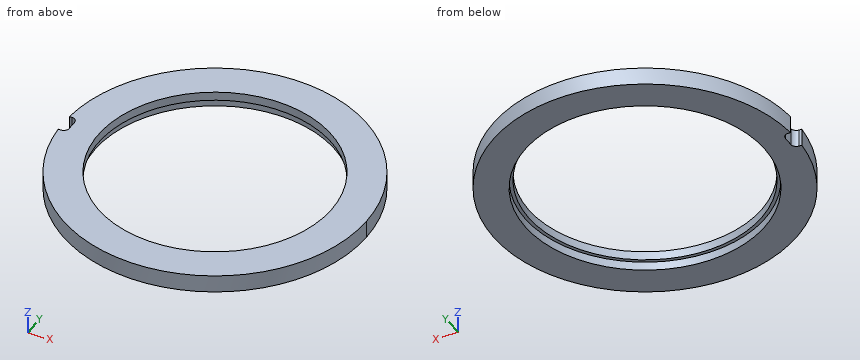
```python
from build123d import *

# Parameters (mm, degrees)
CUT_EXTRUDE_1_DEPTH = 3
FILLET_2_R          = 0.6


with BuildPart() as part:
    # Эскиз1 → Повернуть1 (revolve)
    with BuildSketch(Plane(origin=(0, 0, 0), x_dir=(1, 0, 0), z_dir=(0, 1, 0)), mode=Mode.PRIVATE) as revolve_1_sk:
        Polygon((-16.7, 0), (-12.825, 0), (-12.825, 0.98), (-13.2, 0.98), (-13.2, 1.95), (-16.7, 1.95), align=None)
    revolve(revolve_1_sk.sketch.rotate(Axis((0, 0, 0), (0, 0, -1)), 180), axis=Axis((0, 0, 0), (0, 0, -1)))

    # Эскиз2 → Вырез-Вытянуть1 (cut)
    with BuildSketch(Plane(origin=(0, 0, -1.95), x_dir=(-1, 0, 0), z_dir=(0, 0, -1))):
        with BuildLine():
            Line((16.660357139, 1.15), (15.773622825, 1.15))
            Line((15.773622825, 1.15), (15.773622825, -1.15))
            Line((15.773622825, -1.15), (16.660357139, -1.15))
            ThreePointArc((16.660357139, -1.15), (16.850858655, 0), (16.660357139, 1.15))
        make_face()
    extrude(amount=-CUT_EXTRUDE_1_DEPTH, mode=Mode.SUBTRACT)

    # Скругление2
    fillet_2_edges = [part.edges().sort_by_distance(p)[0] for p in [
        (-15.773622825, -1.15, -0.975),
        (-15.773622825, 1.15, -0.975),
    ]]
    fillet(fillet_2_edges, radius=FILLET_2_R)


solid = part.part
```
Design review of the part built by this model. Coordinates are the model's own, in mm. Coordinates: 2 decimals unless noted, no trailing zeros. Write each loop counter-clockwise with the first axis right and the second up, starting at its lowest first coordinate (ties: lowest second). Pieces come first, ordered by that corner, then holes.
1) To check wall thickness, follow L1, parallel to Y at x = 0, z = -0.6 (3 decimals); L2, parallel to Y at x = 0, z = -1.7; L3, parallel to X at y = 5.5, z = -0.35. State the ranges of each line that lie inside material, in increasing order.
2) Add section B-B (z = -0.55). Write out the cut boundary in (x, y) (3 decimals).
3) Add section C-C (y = -4.5). Write out the cut boundary in (x, z).
4) Add section A-A (x = 0). Write out the cut boundary in (y, z) (3 decimals), plus the area to 3 significant figures.
Check result:
1. L1: y = -16.7 to -12.825, 12.825 to 16.7
1. L2: y = -16.7 to -13.2, 13.2 to 16.7
1. L3: x = -15.77 to -11.59, 11.59 to 15.77
2. outline: (-16.66, -1.15) arc R16.7 ccw (long way) to (-16.66, 1.15) - (-16.374, 1.15) arc R0.6 cw to (-15.774, 0.55) - (-15.774, -0.55) arc R0.6 cw to (-16.374, -1.15) - close; hole circle Ø25.65 at (0, 0)
3. outline: (-16.08, -1.95) - (-12.41, -1.95) - (-12.41, -0.98) - (-12.01, -0.98) - (-12.01, 0) - (-16.08, 0) - close; (12.01, -0.98) - (12.41, -0.98) - (12.41, -1.95) - (16.08, -1.95) - (16.08, 0) - (12.01, 0) - close
4. outline: (-16.7, -1.95) - (-13.2, -1.95) - (-13.2, -0.98) - (-12.825, -0.98) - (-12.825, 0) - (-16.7, 0) - close; (12.825, -0.98) - (13.2, -0.98) - (13.2, -1.95) - (16.7, -1.95) - (16.7, 0) - (12.825, 0) - close
4. area: 14.4 mm2
